Verification items for the finished model (mm, model axes). Face numbers are marked on the shaded views. A direction names the side the tool comes from. Give positions to 0.01 mm unless a question says otherwise; leave off trailing zeros. Loops run counter-clockwise (first coordinate to the right, second up) from the corner with the lowest first, then second, coordinate; pieces in that order, holes last. Notation, with made-up numbers: M 15.25,31 L 37.25,31 A16 cw 37.25,43 Z; hole C 29.5,89.25 d2. An arc over 180 degrees is marked long. Answer in a Markdown table with one row per item.
```python
from build123d import *

# Parameters (mm, degrees)
SCHIZZO1_R                   = 2.75
ESTRUSIONE_ESTRUSIONE1_DEPTH = 4.1
SCHIZZO2_W                   = 9
SCHIZZO2_H                   = 3
ESTRUSIONE_ESTRUSIONE2_DEPTH = 1.5
RACCORDO1_R                  = 0.5
SCHIZZO3_R                   = 2
ESTRUSIONE_ESTRUSIONE3_DEPTH = 4
SCHIZZO4_R                   = 0.75
ESTRUSIONE_ESTRUSIONE4_DEPTH = 1
RIVOLUZIONE1_ANGLE           = 180
ESTRUSIONE_ESTRUSIONE5_DEPTH = 1.5
SCHIZZO7_R                   = 1.5
TAGLIO_ESTRUSIONE2_DEPTH     = 3.1
SCHIZZO8_R                   = 0.5
TAGLIO_ESTRUSIONE5_DEPTH     = 4
ESTRUSIONE_ESTRUSIONE6_DEPTH = 0.3
RACCORDO5_R                  = 0.1


with BuildPart() as part:
    # Schizzo1 → Estrusione-Estrusione1 (new body)
    with BuildSketch(Plane.XY):
        Circle(SCHIZZO1_R)
    extrude(amount=ESTRUSIONE_ESTRUSIONE1_DEPTH)

    # Schizzo2 → Estrusione-Estrusione2 (add)
    with BuildSketch(Plane.XY.offset(4.1)):
        Rectangle(SCHIZZO2_W, SCHIZZO2_H)
    extrude(amount=-ESTRUSIONE_ESTRUSIONE2_DEPTH)

    # Raccordo1
    raccordo1_edges = [part.edges().sort_by_distance(p)[0] for p in [
        (4.5, -1.5, 3.35),
        (-4.5, 1.5, 3.35),
        (4.5, 1.5, 3.35),
        (-4.5, -1.5, 3.35),
    ]]
    fillet(raccordo1_edges, radius=RACCORDO1_R)

    # Schizzo3 → Estrusione-Estrusione3 (add)
    with BuildSketch(Plane.XY.offset(4.1)):
        with Locations((0, 0.5)):
            Circle(SCHIZZO3_R)
    extrude(amount=ESTRUSIONE_ESTRUSIONE3_DEPTH)

    # Schizzo4 → Estrusione-Estrusione4 (add)
    with BuildSketch(Plane.XY.offset(8.1)):
        with Locations((0, -0.5)):
            Circle(SCHIZZO4_R)
    extrude(amount=ESTRUSIONE_ESTRUSIONE4_DEPTH)

    # Schizzo5 → Rivoluzione1 (revolve)
    with BuildSketch(Plane.XY.offset(9.1)):
        with BuildLine():
            Line((0, 0.25), (0, -1.25))
            ThreePointArc((0, -1.25), (0.75, -0.5), (0, 0.25))
        make_face()
    revolve(axis=Axis((0, 0.25, 9.1), (0, -1, 0)), revolution_arc=RIVOLUZIONE1_ANGLE)

    # Schizzo6 → Estrusione-Estrusione5 (add)
    with BuildSketch(Plane.XY):
        with BuildLine():
            Line((-2, -8), (-2, 5))
            ThreePointArc((-2, 5), (0, 5.385164807), (2, 5))
            Line((2, 5), (2, -8))
            ThreePointArc((2, -8), (0, -10), (-2, -8))
        make_face()
    extrude(amount=ESTRUSIONE_ESTRUSIONE5_DEPTH)

    # Schizzo7 → Taglio-Estrusione2 (cut)
    with BuildSketch(Plane(origin=(0, 0, 0), x_dir=(-1, 0, 0), z_dir=(0, 0, -1))):
        with Locations((0, 0.5)):
            Circle(SCHIZZO7_R)
    extrude(amount=-TAGLIO_ESTRUSIONE2_DEPTH, mode=Mode.SUBTRACT)

    # Schizzo8 → Taglio-Estrusione5 (cut)
    with BuildSketch(Plane(origin=(0, 0, 3.1), x_dir=(-1, 0, 0), z_dir=(0, 0, -1))):
        with Locations((0, 0.5)):
            Circle(SCHIZZO8_R)
    extrude(amount=-TAGLIO_ESTRUSIONE5_DEPTH, mode=Mode.SUBTRACT)

    # Schizzo9 → Estrusione-Estrusione6 (add)
    with BuildSketch(Plane(origin=(0, 0, 0), x_dir=(-1, 0, 0), z_dir=(0, 0, -1))):
        with BuildLine():
            Line((-0.5, -9.5), (-0.5, -1.5))
            ThreePointArc((-0.5, -1.5), (0, -1), (0.5, -1.5))
            Line((0.5, -1.5), (0.5, -9.5))
            ThreePointArc((0.5, -9.5), (0, -10), (-0.5, -9.5))
        make_face()
    extrude(amount=ESTRUSIONE_ESTRUSIONE6_DEPTH)

    # Raccordo5
    raccordo5_edges = [part.edges().sort_by_distance(p)[0] for p in [
        (0, -10, -0.3),
        (-0.5, -5.5, -0.3),
        (0, -1, -0.3),
        (0.5, -5.5, -0.3),
    ]]
    fillet(raccordo5_edges, radius=RACCORDO5_R)


solid = part.part
```
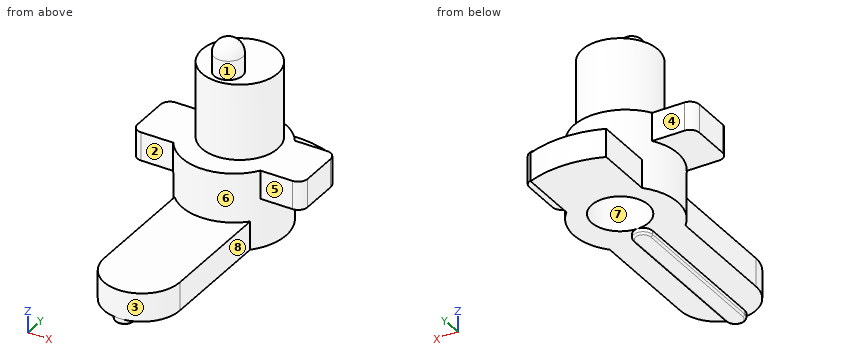
Item 1: Go/stop test with flat-tipped pins: pin 1 (4 mm diameter, centred on x = -1, y = 4.5, fed in from +Z); pin 2 (1.2 mm diameter, centred on x = 0.5, y = -6, fed in from +Z); pin 3 (2 mm diameter, centred on x = -1, y = 1, fed in from +Z). Record where each tip stops, or that it passes through.
Reported:
| item | result |
|---|---|
| pin 1 | stops at z = 4.1 |
| pin 2 | stops at z = 1.5 |
| pin 3 | stops at z = 8.1 |
Item 2: Sectioned sample at C-C (z = 5.5). Record the cut outline in (x, y), and give its area (3 significant figures).
Reported:
| item | result |
|---|---|
| outline | C 0,0.5 d4; hole C 0,0.5 d1 |
| area | 11.8 mm^2 |
Item 3: Sectioned sample at B-B (y = -0.5). Record the cut outline in (x, z).
Reported:
| item | result |
|---|---|
| outline | M -4.5,2.6 L -2.7,2.6 L -2.7,0 L -1.12,0 L -1.12,3.1 L 1.12,3.1 L 1.12,0 L 2.7,0 L 2.7,2.6 L 4.5,2.6 L 4.5,4.1 L 1.73,4.1 L 1.73,8.1 L 0.75,8.1 L 0.75,9.1 A0.75 ccw -0.75,9.1 L -0.75,8.1 L -1.73,8.1 L -1.73,4.1 L -4.5,4.1 Z |
Item 4: Tool access check on the marked faces 1, 2, 3, 4 and 5. Record the directions out of +Z, -Z, +X, -X, +Y, -Y that give a thin tool (end or side, any length) a straight path to the whole face; none if there is none.
Reported:
| item | result |
|---|---|
| face 1 | +Z |
| face 2 | +Z, -Z, -X, -Y |
| face 3 | +Z, -Z, -Y |
| face 4 | +Z, -Z, -X, +Y |
| face 5 | +Z, -Z, +X, -Y |
Item 5: Sectioned sample at D-D (x = 3). Record the cut outline in (y, z), and give its area (3 significant figures).
Reported:
| item | result |
|---|---|
| outline | M -1.5,2.6 L 1.5,2.6 L 1.5,4.1 L -1.5,4.1 Z |
| area | 4.50 mm^2 |
Item 6: Sectioned sample at A-A (z = 1). Record the cut outline in (x, y).
Reported:
| item | result |
|---|---|
| outline | M -2,-8 A2 ccw 2,-8 L 2,-1.89 A2.75 ccw 2,1.89 L 2,5 A5.39 ccw -2,5 L -2,1.89 A2.75 ccw -2,-1.89 Z; hole C 0,0.5 d3 |
Item 7: Scan lines: L1, parallel to Y at x = 0, z = 1.6; L2, parallel to Y at x = 0, z = 5.3; L3, parallel to Z at x = 1.25, y = -7.25. Record each from-to range of solid material in increasing order. Write a range as [from, to].
Reported:
| item | result |
|---|---|
| L1 | y = [-2.75, -1], [2, 2.75] |
| L2 | y = [-1.5, 0], [1, 2.5] |
| L3 | z = [0, 1.5] |
Item 8: Release check for a two-part mould opening along Y. For the marked faces 6, 7 and 8 record: released by +Y, released by -Y, zero draft, split by the parting line, or undercut.
Reported:
| item | result |
|---|---|
| face 6 | split by the parting line |
| face 7 | undercut |
| face 8 | zero draft |
